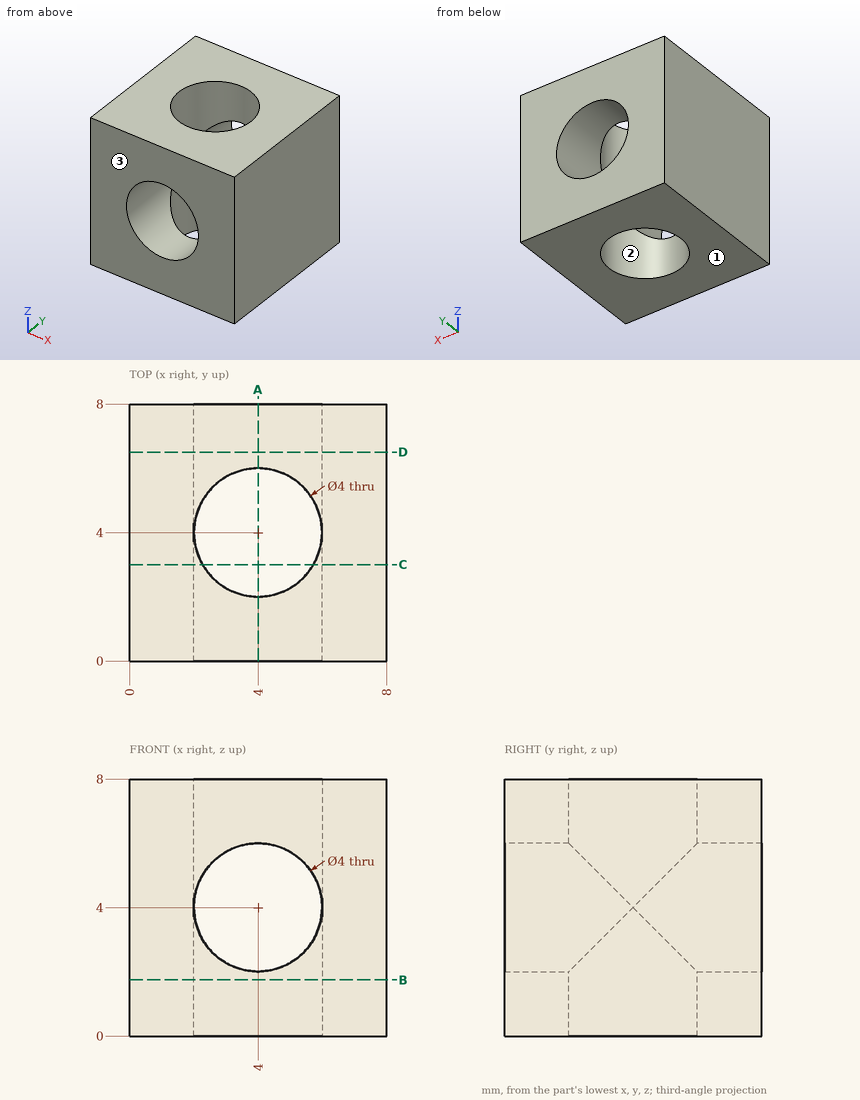
The figure shows three views and two pictorial views of one solid part (mm, origin at its lowest corner). Answer the questions. Coordinates: 2 decimals unless noted, no trailing zeros. Loops run counter-clockwise (first coordinate to the right, second up) from the corner with the lowest first, then second, coordinate; pieces in that order, holes last. Notation, with made-up numbers: (52, 32) - (86, 32) arc R28 ccw to (86, 64) - close; hole circle Ø8 at (62.5, 72). An arc over 180 degrees is marked (long way). Use a Markdown table: item, result. Add a question column.
1) The part is cut by section B-B, the plane z = 1.75. Give the vertices of the cut face in (x, y), and give its area (3 significant figures).
2) The part is cut by section A-A, the plane x = 4. Give the vertices of the cut face in (y, z).
3) The mould has two halves that part along Y. Classify the marked faces 1, 2 and 3: released by +Y, released by -Y, zero draft, split by the parting line, or undercut.
4) The part is cut by section C-C, the plane y = 3. Give the vertices of the cut face in (x, z).
5) Find the intervals of material crossed by line 1 (Z direction, x = 4, y = 1.25); line 2 (X direction, y = 2.75, z = 5.75), in increasing order.
Here are the results:
| question | item | result |
|---|---|---|
| 1 | outline | (0, 0) - (8, 0) - (8, 8) - (0, 8) - close; hole circle Ø4 at (4, 4) |
| 1 | area | 51.4 mm^2 |
| 2 | outline | (0, 0) - (2, 0) - (2, 2) - (0, 2) - close; (0, 6) - (2, 6) - (2, 8) - (0, 8) - close; (6, 0) - (8, 0) - (8, 2) - (6, 2) - close; (6, 6) - (8, 6) - (8, 8) - (6, 8) - close |
| 3 | face 1 | zero draft |
| 3 | face 2 | undercut |
| 3 | face 3 | released by -Y |
| 4 | outline | (0, 0) - (2.27, 0) - (2.27, 3) arc R2 cw to (2.27, 5) - (2.27, 8) - (0, 8) - close; (5.73, 0) - (8, 0) - (8, 8) - (5.73, 8) - (5.73, 5) arc R2 cw to (5.73, 3) - close |
| 5 | line 1 | z = 0 to 2, 6 to 8 |
| 5 | line 2 | x = 0 to 2.44, 5.56 to 8 |
